from build123d import *

# Parameters (mm, degrees)
SKETCH1_R           = 1
BOSS_EXTRUDE1_DEPTH = 3


with BuildPart() as part:
    # Sketch1 → Boss-Extrude1 (new body)
    with BuildSketch(Plane(origin=(0, 0, 0), x_dir=(1, 0, 0), z_dir=(0, 1, 0))):
        Polygon((2.020725942, 3.5), (-2.020725942, 3.5), (-4.041451884, 0), (-2.020725942, -3.5), (2.020725942, -3.5), (4.041451884, 0), align=None)
        Circle(SKETCH1_R, mode=Mode.SUBTRACT)
    extrude(amount=BOSS_EXTRUDE1_DEPTH)

    # Sketch2 → Revolve1 (revolve)
    with BuildSketch(Plane.XY):
        Polygon((2.5, 3), (1, 3), (1, 10.5), (3, 10.5), (3, 4.5), (2.5, 4.5), align=None)
        Polygon((1, 0), (1.900415076, 0), (0.5, -2), (0.2, -2), align=None)
    revolve(axis=Axis((0, -2, 0), (0, 1, 0)))


solid = part.part
Can you work these out from the model? Positions are in its coordinate system, mm. A direction names the side the tool comes from. Give positions to 0.01 mm unless a question says otherwise; leave off trailing zeros. Loops run counter-clockwise (first coordinate to the right, second up) from the corner with the lowest first, then second, coordinate; pieces in that order, holes last. Notation, with made-up numbers: (27, 11) - (48, 11) arc R16 cw to (48, 26) - close; hole circle Ø5 at (70.25, 5). An arc over 180 degrees is marked (long way). One line per item, written item: value.
(1) If we section it at B-B, the plane y = 1.75: List the corners of the cut face in (x, z) for me, plus the area to 3 significant figures.
Verdict:
outline: (-4.04, 0) - (-2.02, -3.5) - (2.02, -3.5) - (4.04, 0) - (2.02, 3.5) - (-2.02, 3.5) - close; hole circle Ø2 at (0, 0)
area: 39.3 mm^2
(2) If we section it at D-D, the plane x = 3.75: List the corners of the cut face in (y, z) for me.
Verdict:
outline: (0, -0.5) - (3, -0.5) - (3, 0.5) - (0, 0.5) - close
(3) I'm going to push flat-ended pins straight in: pin 1 (1.8 mm diameter, centred on x = -0.5, z = 1.5, fed in from -Y); pin 2 (1 mm diameter, centred on x = -3, z = 1.5, fed in from -Y); pin 3 (4 mm diameter, centred on x = 3, y = 8.5, fed in from +Z). Where does each tip first touch, or does it pass through?
Verdict:
pin 1: y = -1.74
pin 2: y = 0
pin 3: z = 2.83
(4) If we section it at C-C, the plane y = 5.5: List the corners of the cut face in (x, z) for me.
Verdict:
outline: circle Ø6 at (0, 0); hole circle Ø2 at (0, 0)
(5) If we section it at A-A, the plane x = 0: List the corners of the cut face in (y, z) for me.
Verdict:
outline: (-2, -0.5) - (0, -1.9) - (0, -3.5) - (3, -3.5) - (3, -2.5) - (4.5, -2.5) - (4.5, -3) - (10.5, -3) - (10.5, -1) - (0, -1) - (-2, -0.2) - close; (-2, 0.2) - (0, 1) - (10.5, 1) - (10.5, 3) - (4.5, 3) - (4.5, 2.5) - (3, 2.5) - (3, 3.5) - (0, 3.5) - (0, 1.9) - (-2, 0.5) - close
(6) On a 3-axis mill with a long thin cutter (end or side, diameter ignored), from which of +Z, -Z, +X, -X, +Y, -Y can I reach the whole of each face in a straight line? I mean faces 4 (the face through (3, 3, 0)), 5 (the face through (0, 1, 3.5)), 6 (the face through (0, 5, 1)). Say none if no direction works.
Verdict:
face 4: none
face 5: +Z, +X, -X, +Y, -Y
face 6: +Y
(7) I need wall thicknesses on line 1 along X through (y, z) = (3.25, 0); line 2 along Z through (x, y) = (0, 5.75). Which ranges of each line are inside material? Lowest first, please.
Verdict:
line 1: -2.5 to -1, 1 to 2.5
line 2: -3 to -1, 1 to 3
(8) If we mould it in two halves opening along Y, with no side actions, what happens to faces 1 (the face through (3, 1.5, 1.8)), 2 (the face through (2, 0, -1)), 3 (the face through (-0.54, 3.74, 2.44))? For each: released by +Y, released by -Y, zero draft, split by the parting line, or undercut.
Verdict:
face 1: zero draft
face 2: released by -Y
face 3: undercut
